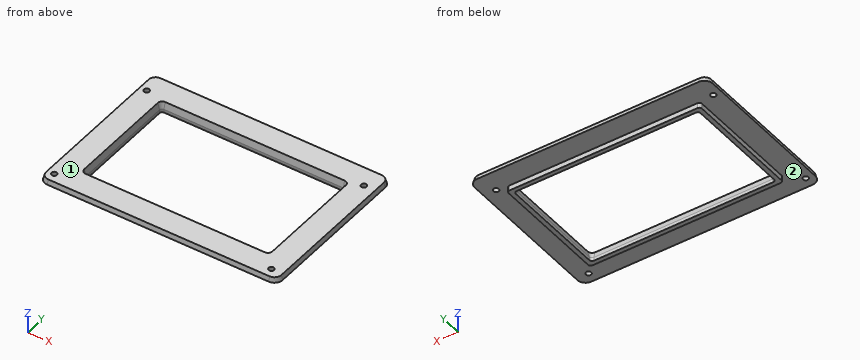
from build123d import *

# Parameters (mm, degrees)
SKETCH1_W                    = 139.7
SKETCH1_H                    = 96.266
BOSS_EXTRUDE1_DEPTH          = 2.794
F_1_8_0_125_DIAMETER_HOLE1_D = 3.175
SKETCH4_W                    = 107.9999999
SKETCH4_H                    = 64.79999994
CUT_EXTRUDE1_DEPTH           = 85.874110452
FILLET1_R                    = 1.524
FILLET2_R                    = 5.08
BOSS_EXTRUDE2_START          = 3.048
SKETCH5_W                    = 113.0799999
SKETCH5_H                    = 69.75759988
BOSS_EXTRUDE2_DEPTH          = 3.048
FILLET3_R                    = 1.524
CHAMFER1_SIZE                = 1.016
CHAMFER1_SIZE2               = 3.79176362
CHAMFER2_SIZE                = 1.016
CHAMFER2_SIZE_2              = 3.79176362


with BuildPart() as part:
    # Sketch1 → Boss-Extrude1 (new body)
    with BuildSketch(Plane.XY):
        Rectangle(SKETCH1_W, SKETCH1_H)
    extrude(amount=BOSS_EXTRUDE1_DEPTH)

    # 1/8 (0.125) Diameter Hole1 (through all)
    with Locations(Plane.XY.offset(2.794)):
        with Locations((-64.82, -41.975), (-64.82, 35.625), (62.28, -41.975), (62.28, 35.625)):
            Hole(F_1_8_0_125_DIAMETER_HOLE1_D / 2)

    # Sketch4 → Cut-Extrude1 (cut, through all)
    with BuildSketch(Plane.XY.offset(2.794)):
        with Locations((0, 0.06120003)):
            Rectangle(SKETCH4_W, SKETCH4_H)
    extrude(amount=-CUT_EXTRUDE1_DEPTH, mode=Mode.SUBTRACT)

    # Fillet1
    fillet1_edges = [part.edges().sort_by_distance(p)[0] for p in [
        (53.99999995, 32.4612, 1.397),
        (53.99999995, -32.33879994, 1.397),
        (-53.99999995, -32.33879994, 1.397),
        (-53.99999995, 32.4612, 1.397),
    ]]
    fillet(fillet1_edges, radius=FILLET1_R)

    # Fillet2
    fillet2_edges = [part.edges().sort_by_distance(p)[0] for p in [
        (69.85, -48.133, 1.397),
        (-69.85, -48.133, 1.397),
        (-69.85, 48.133, 1.397),
        (69.85, 48.133, 1.397),
    ]]
    fillet(fillet2_edges, radius=FILLET2_R)

    # Sketch5 → Boss-Extrude2 (add)
    with BuildSketch(Plane(origin=(0, 0, 0), x_dir=(-1, 0, 0), z_dir=(0, 0, -1)).offset(BOSS_EXTRUDE2_START)):
        Rectangle(SKETCH5_W, SKETCH5_H)
        with BuildLine():
            Line((-53.99999995, -30.81479994), (-53.99999995, 30.9372))
            ThreePointArc((-53.99999995, 30.9372), (-53.553630685, 32.014830735), (-52.47599995, 32.4612))
            Line((-52.47599995, 32.4612), (52.47599995, 32.4612))
            ThreePointArc((52.47599995, 32.4612), (53.553630685, 32.014830735), (53.99999995, 30.9372))
            Line((53.99999995, 30.9372), (53.99999995, -30.81479994))
            ThreePointArc((53.99999995, -30.81479994), (53.553630685, -31.892430675), (52.47599995, -32.33879994))
            Line((52.47599995, -32.33879994), (-52.47599995, -32.33879994))
            ThreePointArc((-52.47599995, -32.33879994), (-53.553630685, -31.892430675), (-53.99999995, -30.81479994))
        make_face(mode=Mode.SUBTRACT)
    extrude(amount=-BOSS_EXTRUDE2_DEPTH)

    # Fillet3
    fillet3_edges = [part.edges().sort_by_distance(p)[0] for p in [
        (-56.53999995, -34.87879994, -1.524),
        (-56.53999995, 34.87879994, -1.524),
        (56.53999995, 34.87879994, -1.524),
        (56.53999995, -34.87879994, -1.524),
    ]]
    fillet(fillet3_edges, radius=FILLET3_R)

    # Chamfer1
    chamfer1_edges = [part.edges().sort_by_distance(p)[0] for p in [
        (0, -32.33879994, 2.794),
        (-53.99999995, 0.06120003, 2.794),
        (53.99999995, 0.06120003, 2.794),
        (0, 32.4612, 2.794),
        (-53.553630685, -31.892430675, 2.794),
        (53.553630685, -31.892430675, 2.794),
        (53.553630685, 32.014830735, 2.794),
        (-53.553630685, 32.014830735, 2.794),
    ]]
    chamfer1_side = [part.faces().sort_by_distance(p)[0] for p in [
        (0, -46.436437807, 2.794),
    ]]
    chamfer(chamfer1_edges, length=CHAMFER1_SIZE, length2=CHAMFER1_SIZE2, reference=chamfer1_side[0])

    # Chamfer2
    # the kernel refuses this chamfer: 3.79176362, 1.016 mm, written as the material it takes off along each edge
    with BuildSketch(Plane(origin=(-69.85, 43.053, 2.794), x_dir=(0.9905000388259543, 0, 0.13751244702129017), z_dir=(0, -1, 0)), Plane(origin=(69.85, -43.053, 2.794), x_dir=(-0.9905000388259543, 0, 0.13751244702129017), z_dir=(0, 1, 0))) as chamfer2_piece_1:
        Polygon((CHAMFER2_SIZE * 0.990500038826, -CHAMFER2_SIZE * 0.137512447021), (-CHAMFER2_SIZE_2 * 0.137512447039, -CHAMFER2_SIZE_2 * 0.990500038954), (0, 0), align=None)
    extrude(amount=86.106, mode=Mode.SUBTRACT)
    with BuildSketch(Plane(origin=(-64.77, -43.053, 2.794), x_dir=(0, -1, 0), z_dir=(1, 0, 0))) as chamfer2_piece_2:
        Polygon((5.08 - CHAMFER2_SIZE, 0), (5.08, CHAMFER2_SIZE_2), (5.08, 0), align=None)
    revolve(axis=Axis((-64.77, -43.053, 2.794), (0, 0, -1)), revolution_arc=90, mode=Mode.SUBTRACT)
    with BuildSketch(Plane(origin=(-64.77, -48.133, 2.794), x_dir=(0, 0.990500038825954, 0.13751244702129148), z_dir=(1, 0, 0)), Plane(origin=(64.77, 48.133, 2.794), x_dir=(0, -0.990500038825954, 0.13751244702129148), z_dir=(-1, 0, 0))) as chamfer2_piece_3:
        Polygon((CHAMFER2_SIZE * 0.990500038826, -CHAMFER2_SIZE * 0.137512447021), (-CHAMFER2_SIZE_2 * 0.137512447039, -CHAMFER2_SIZE_2 * 0.990500038954), (0, 0), align=None)
    extrude(amount=129.54, mode=Mode.SUBTRACT)
    with BuildSketch(Plane(origin=(64.77, -43.053, 2.794), x_dir=(0, -1, 0), z_dir=(-1, 0, 0))) as chamfer2_piece_4:
        Polygon((5.08 - CHAMFER2_SIZE, 0), (5.08, -CHAMFER2_SIZE_2), (5.08, 0), align=None)
    revolve(axis=Axis((64.77, -43.053, 2.794), (0, 0, 1)), revolution_arc=90, mode=Mode.SUBTRACT)
    with BuildSketch(Plane(origin=(64.77, 43.053, 2.794), x_dir=(1, 0, 0), z_dir=(0, -1, 0))) as chamfer2_piece_5:
        Polygon((5.08 - CHAMFER2_SIZE, 0), (5.08, -CHAMFER2_SIZE_2), (5.08, 0), align=None)
    revolve(axis=Axis((64.77, 43.053, 2.794), (0, 0, 1)), revolution_arc=90, mode=Mode.SUBTRACT)
    with BuildSketch(Plane(origin=(-64.77, 43.053, 2.794), x_dir=(-1, 0, 0), z_dir=(0, -1, 0))) as chamfer2_piece_6:
        Polygon((5.08 - CHAMFER2_SIZE, 0), (5.08, CHAMFER2_SIZE_2), (5.08, 0), align=None)
    revolve(axis=Axis((-64.77, 43.053, 2.794), (0, 0, -1)), revolution_arc=90, mode=Mode.SUBTRACT)


solid = part.part
Work out the finished part from the listing and answer in its coordinate system (mm). Face numbers are marked on the shaded views. A direction names the side the tool comes from. Give positions to 0.01 mm unless a question says otherwise; leave off trailing zeros. Order: outer loops, then holes, each group sorted by start corner. A loop starts at its lowest first (then second) coordinate and runs counter-clockwise, first axis right, second up. Notation, with made-up numbers: (63, 80) -> (84, 80) arc R15 cw to (84, 108) -> close; hole circle Ø10 at (-8, 37.5). An arc over 180 degrees is marked (long way). One line per item, written item: value.
Item 1: Straight lines are drawn through the part: probe 1 along X at (y, z) = (8, -2.55); probe 2 along Y at (x, z) = (-9.5, -2.5); probe 3 along Y at (x, z) = (-64.82, 1.7). For each, find the intervals that lie inside material, in ascending order.
Answer sheet:
probe 1: -56.54 to -54, 54 to 56.54
probe 2: -34.88 to -32.34, 32.46 to 34.88
probe 3: -47.41 to -43.56, -40.39 to 34.04, 37.21 to 47.41
Item 2: Find section C-C, the plane x = 62.28. Give the vertices of the cut face in (y, z), plus the area to 3 significant figures.
Answer sheet:
outline: (-47.87, 0) -> (-43.56, 0) -> (-43.56, 2.79) -> (-47.12, 2.79) -> close; (-40.39, 0) -> (34.04, 0) -> (34.04, 2.79) -> (-40.39, 2.79) -> close; (37.21, 0) -> (47.87, 0) -> (47.12, 2.79) -> (37.21, 2.79) -> close
area: 248 mm²
Item 3: Find section B-B, the plane y = 10. Give the vertices of the cut face in (x, z).
Answer sheet:
outline: (-69.58, 0) -> (-56.54, 0) -> (-56.54, -3.05) -> (-54, -3.05) -> (-54, -1) -> (-55.02, 2.79) -> (-68.83, 2.79) -> close; (54, -3.05) -> (56.54, -3.05) -> (56.54, 0) -> (69.58, 0) -> (68.83, 2.79) -> (55.02, 2.79) -> (54, -1) -> close
Item 4: Find section D-D, the plane z = 1.6. Give the vertices of the cut face in (x, y) (1 decimal), plus the area to 3 significant figures.
Answer sheet:
outline: (-69.2, -43.1) arc R4.4 ccw to (-64.8, -47.4) -> (64.8, -47.4) arc R4.4 ccw to (69.2, -43.1) -> (69.2, 43.1) arc R4.4 ccw to (64.8, 47.4) -> (-64.8, 47.4) arc R4.4 ccw to (-69.2, 43.1) -> close; hole circle Ø3.2 at (-64.8, -42); hole circle Ø3.2 at (-64.8, 35.6); hole (-54.7, -30.8) arc R2.2 ccw to (-52.5, -33) -> (52.5, -33) arc R2.2 ccw to (54.7, -30.8) -> (54.7, 30.9) arc R2.2 ccw to (52.5, 33.2) -> (-52.5, 33.2) arc R2.2 ccw to (-54.7, 30.9) -> close; hole circle Ø3.2 at (62.3, -42); hole circle Ø3.2 at (62.3, 35.6)
area: 5,840 mm²
Item 5: Find section A-A, the plane x = -16. Give the vertices of the cut face in (y, z), plus the area to 3 significant figures.
Answer sheet:
outline: (-47.87, 0) -> (-34.88, 0) -> (-34.88, -3.05) -> (-32.34, -3.05) -> (-32.34, -1) -> (-33.35, 2.79) -> (-47.12, 2.79) -> close; (32.46, -3.05) -> (34.88, -3.05) -> (34.88, 0) -> (47.87, 0) -> (47.12, 2.79) -> (33.48, 2.79) -> (32.46, -1) -> close
area: 95.6 mm²
Item 6: Flat-ended cylindrical pins translate along their axes: P1, Ø4, axis at x = 62.28, y = 35.625, coming from the -Z side; P2, Ø3.5, axis at x = 13.5, z = -2, coming from the -Y side; P3, Ø0.9, axis at y = 12.5, z = -1, coming from the -X side. Find the tip coordinate at first contact, or state that the pin passes through.
Answer sheet:
P1: z = 0
P2: y = -34.88
P3: x = -56.54
Item 7: A tool of negligible diameter and unlimited length cuts with its end or side. For the marked faces 1 and 2, from which of +Z, -Z, +X, -X, +Y, -Y can it reach the whole face along a straight path? Write none if from no direction.
Answer sheet:
face 1: +Z, +X, -X, +Y, -Y
face 2: -Z
